Source: CAD feature listing. Evaluate the final solid. Frame: model axes, mm. A direction names the side the tool comes from. Coordinates: 2 decimals unless noted, no trailing zeros. Order: outer loops, then holes, each group sorted by start corner. A loop starts at its lowest first (then second) coordinate and runs counter-clockwise, first axis right, second up. Notation, with made-up numbers: (5.5, 32.5) -> (55.5, 32.5) arc R20 ccw to (55.5, 37.5) -> close; hole circle Ø3 at (-12, 39). An arc over 180 degrees is marked (long way). Put each result on its own line as item: value.
Autodesk Inventor part; units mm, degrees
ref_plane "YZ Plane" through (0, 0, 0) normal (1, 0, 0) x (0, 1, 0)
ref_plane "XZ Plane" through (0, 0, 0) normal (0, 1, 0) x (-1, 0, 0)
ref_plane "XY Plane" through (0, 0, 0) normal (0, 0, 1) x (1, 0, 0)
sketch "Sketch1" plane through (0, 0, 0) normal (0, 1, 0) x (-1, 0, 0)
  line L0 (52, -10) -> (52, 16)
  arc A0 (52, 16) -> (51, 17) centre (51, 16) ccw
  line L1 (51, 17) -> (-22, 17)
  arc A1 (50, -10) -> (51, -9) centre (51, -10) ccw
  line L2 (-22, 17) -> (-22, -11)
  line L3 (-2, 20) -> (-19, 20)
  line L4 (-1, 5) -> (-1, 14)
  line L5 (0, 14) -> (0, 5)
  line L6 (-1, 1) -> (-1, -8)
  line L7 (51, 16) -> (-21, 16)
  line L8 (51, -2) -> (51, 8)
  line L9 (52, 8) -> (52, -2)
  line L10 (51, -10) -> (-21, -10)
  line L11 (51, 8) -> (52, 8)
  line L12 (52, 8) -> (52, -2)
  line L13 (52, -2) -> (51, -2)
  line L14 (51, -2) -> (51, 8)
  line L15 (51, -10) -> (51, 16)
  line L16 (52, 16) -> (52, -10)
  line L17 (51, -11) -> (-22, -11)
  line L18 (-21, 16) -> (-21, -10)
  line L19 (-2, 20) -> (1, 17)
  line L20 (-2, 20) -> (2.6568, 20) construction
  line L21 (-22, 17) -> (-19, 20)
  line L22 (-22, 17) -> (-5.0328, 17) construction
  line L23 (-1, 1) -> (0.3284, 1)
  line L24 (0.3284, 1) -> (0.3284, -8)
  line L25 (0.3284, -8) -> (-1, -8)
  line L26 (-1, -8) -> (-1, 1)
  line L27 (-1, 14) -> (0, 14)
  line L28 (0, 14) -> (0, 5)
  line L29 (0, 5) -> (-1, 5)
  line L30 (-1, 5) -> (-1, 14)
  point P0 (0, 0)
  dimension "d0" = 45
  dimension "d1" = 45
extrude "Extrusion1" add sketch "Sketch1" against normal blind 2 contours A1 L15 L13 L0 | A1 L10 L15 | L13 L8 L11 L0 | L17 L2 L1 A0 L0 L11 L15 L7 L18 L10 A1 | L15 L10 L18 L7 L8 | L21 L3 L19 L1 | L4 L27 L5 L29 | L23 L24 L25 L6
extrude "Extrusion2" add sketch "Sketch1" along normal blind 9 contours A1 L15 L13 L0 | A1 L10 L15 | L13 L8 L11 L0 | L17 L2 L1 A0 L0 L11 L15 L7 L18 L10 A1 | L21 L3 L19 L1
extrude "Extrusion3" add sketch "Sketch1" along normal blind 14 contours A1 L15 L13 L0 | A1 L10 L15 | L17 L2 L1 A0 L0 L11 L15 L7 L18 L10 A1 | L21 L3 L19 L1
sketch "Sketch2" plane through (0, 0, 0) normal (0, 1, 0) x (1, 0, 0)
  line L0 (-51, 10) -> (21, 10)
  line L1 (21, -16) -> (-51, -16)
  line L2 (21, 10) -> (-51, 10)
  line L3 (0, -16) -> (-5, -16)
  line L4 (-5, -16) -> (-5, -11)
  line L5 (-5, -11) -> (0, -11)
  line L6 (0, -11) -> (0, -16)
  line L7 (0, 10) -> (-5, 10)
  line L8 (-5, 10) -> (-5, 5)
  line L9 (-5, 5) -> (0, 5)
  line L10 (0, 5) -> (0, 10)
  line L11 (-5, 10) -> (-35, 10)
  line L12 (-35, 10) -> (-35, 7.5)
  line L13 (-35, 7.5) -> (-5, 7.5)
  line L14 (-5, 7.5) -> (-5, 10)
  line L15 (-51, 2) -> (-51, 10)
  line L16 (-5, -13.5) -> (-51, -13.5)
  line L17 (-51, -13.5) -> (-51, -16)
  line L18 (-51, -16) -> (-5, -16)
  line L19 (-5, -16) -> (-5, -13.5)
  point P0 (0, 0)
  dimension "d8" = 5
  dimension "d9" = 5
  dimension "d10" = 5
  dimension "d11" = 5
  dimension "d12" = 16
extrude "Extrusion4" add sketch "Sketch2" along normal blind 10
sketch "Sketch3" plane through (2, -2, 20) normal (0, 0, 1) x (1, 0, 0)
  line L0 (17, 0) -> (17, 16)
  line L1 (0, 16) -> (17, 2)
  circle A0 centre (8.5, 9) radius 3
  point P0 (-2, 2)
  dimension "d15" = 6
sketch "Sketch4" plane through (0, 0, 0) normal (0, 1, 0) x (1, 0, 0)
  line L0 (0, -16) -> (21, -16)
  line L1 (-51, 10) -> (21, 10)
  line L2 (0, -16) -> (2.5, -16)
  line L3 (2.5, -16) -> (2.5, 10)
  line L4 (2.5, 10) -> (0, 10)
  line L5 (0, 10) -> (0, -16)
  line L6 (2.5, -8) -> (0, -8)
  line L7 (0, -8) -> (0, 2)
  line L8 (0, 2) -> (2.5, 2)
  line L9 (2.5, 2) -> (2.5, -8)
  line L10 (2.5, 2) -> (0, 2)
  line L11 (0, 2) -> (0, 10)
  line L12 (0, 10) -> (2.5, 10)
  line L13 (2.5, 10) -> (2.5, 2)
  line L14 (0, -8) -> (2.5, -8)
  line L15 (2.5, -8) -> (2.5, -16)
  line L16 (2.5, -16) -> (0, -16)
  line L17 (0, -16) -> (0, -8)
  point P0 (0, 0)
  dimension "d16" = 2.5
  dimension "d17" = 8
  dimension "d18" = 8
extrude "Extrusion5" add sketch "Sketch4" along normal blind 14 contours L5 L6 L3 L0 | L5 L1 L3 L8
extrude "Extrusion6" cut sketch "Sketch3" against normal blind 14
sketch "Sketch5" plane through (0, 10, 0) normal (0, 1, 0) x (1, 0, 0)
  line L0 (-35, 10) -> (0, 10)
  line L1 (-35, 10) -> (-35, 7.5)
  line L2 (-35, 7.5) -> (-5, 7.5)
  line L3 (-5, 7.5) -> (-5, 5)
  line L4 (-5, 5) -> (0, 5)
  line L5 (0, 5) -> (0, 10)
  line L6 (0, -16) -> (-51, -16)
  line L7 (0, -16) -> (0, -11)
  line L8 (0, -11) -> (-5, -11)
  line L9 (-5, -11) -> (-5, -13.5)
  line L10 (-5, -13.5) -> (-51, -13.5)
  line L11 (-51, -16) -> (-51, -13.5)
  line L12 (-5, -11) -> (0, -16)
  line L13 (0, 5) -> (0, 10)
  line L14 (0, 10) -> (-5, 5)
  point P0 (0, 0)
  point P1 (-2.5, 7.5)
  point P2 (-2.5, -13.5)
hole "Hole1" at (-2.5, 10, -7.5) at (-2.5, 10, 13.5) direction (0, -1, 0) diameter 2 depth 8 tip angle 118
properties part number "ttgo_lora_oled_case"
1. Cut plane B-B on y = 7. Count the separate pieces of the cut face and the enclosed holes in it, plus the area to 3 significant figures.
Numbers:
separate pieces: 1
enclosed holes: 2
area: 509 mm2
2. Pull-direction query (X, two-part tool) for faces 1 (the flat face through (-52, 6, 3)), 2 (the flat face through (2, 14, 9)), 3 (the flat face through (-5, 5, 12)); classes: pulls with the +X half, pulls with the -X half, needs draft (parallel to the pull), parting line crosses it, or undercut.
Numbers:
face 1: pulls with the -X half
face 2: needs draft
face 3: undercut
3. Cut plane C-C on z = 2.5. Output: boundary loops of the cut face in (x, y).
Numbers:
outline: (-52, -2) -> (22, -2) -> (22, 14) -> (21, 14) -> (21, 0) -> (-51, 0) -> (-51, 9) -> (-52, 9) -> close
4. Set-up query: faces 4 (the flat face through (-15, 6, -11)), 5 (the flat face through (-51, 7, 3)). Return all of +Z, -Z, +X, -X, +Y, -Y with unobstructed straight access to the full face (end or side cutting, diameter ignored); none if empty.
Numbers:
face 4: -Z, +X, -X, +Y, -Y
face 5: +Y
5. Cut plane D-D on x = -8. Output: boundary loops of the cut face in (y, z).
Numbers:
outline: (-2, -11) -> (14, -11) -> (14, -10) -> (10, -10) -> (10, -7.5) -> (0, -7.5) -> (0, 13.5) -> (10, 13.5) -> (10, 16) -> (14, 16) -> (14, 17) -> (-2, 17) -> close
6. Cut plane A-A on x = 10.5. Output: boundary loops of the cut face in (y, z), plus the area to 3 significant figures.
Numbers:
outline: (-2, -11) -> (14, -11) -> (14, -10) -> (0, -10) -> (0, 16) -> (4, 16) -> (4, 20) -> (-2, 20) -> close; (10, 16) -> (14, 16) -> (14, 20) -> (10, 20) -> close
area: 108 mm2
7. Ray query, line 1 along X through (y, z) = (6, -9); line 2 along X through (y, z) = (11.5, 9.5); line 3 along Z through (x, y) = (-2.5, 4.75). Return the intervals inside material, ascending.
Numbers:
line 1: x = -52 to -51, -35 to 2.5, 21 to 22
line 2: x = -52 to -51, 0 to 2.5, 21 to 22
line 3: z = -11 to -8.5, -6.5 to -5, 11 to 12.5, 14.5 to 17
8. First-contact query: pin 1 (3 mm diameter, centred on x = -2.5, z = -7.5, fed in from +Y); pin 2 (8 mm diameter, centred on x = -8.5, y = 2, fed in from +Z). Flat tips, straight axial feed; report the tip coordinate or a pass-through.
Numbers:
pin 1: stops at y = 10
pin 2: stops at z = 17
